Design review of the part built by this model. Coordinates are the model's own, in mm. A direction names the side the tool comes from. Coordinates: 2 decimals unless noted, no trailing zeros. Write each loop counter-clockwise with the first axis right and the second up, starting at its lowest first coordinate (ties: lowest second). Pieces come first, ordered by that corner, then holes.
```python
from build123d import *

# Parameters (mm, degrees)
SKETCH1_W                       = 40.894
SKETCH1_H                       = 25.4
REVOLVE1_ANGLE                  = 180
BOSS_EXTRUDE1_REACH             = 27.4
SKETCH3_W                       = 25.654
SKETCH3_H                       = 4.572
BOSS_EXTRUDE1_DIRECTION_2_REACH = 27.4
SKETCH4_W                       = 25.654
SKETCH4_H                       = 24.524924672
CUT_EXTRUDE1_DEPTH              = 4.572
SKETCH5_W                       = 3.81
SKETCH5_H                       = 2.032
BOSS_EXTRUDE2_DEPTH             = 25.654


with BuildPart() as part:
    # Sketch1 → Revolve1 (revolve)
    with BuildSketch(Plane(origin=(0, 0, 0), x_dir=(1, 0, 0), z_dir=(0, 1, 0))):
        with Locations((20.447, -12.7)):
            Rectangle(SKETCH1_W, SKETCH1_H)
    revolve(axis=Axis((0, 0, 0), (1, 0, 0)), revolution_arc=REVOLVE1_ANGLE)

    # Sketch2 → Cut-Revolve1 (revolve, cut)
    with BuildSketch(Plane(origin=(0, 0, 0), x_dir=(1, 0, 0), z_dir=(0, 1, 0))):
        Polygon((0, 0), (41.402, 0), (41.402, -20.701), (40.132, -20.701), (1.27, -20.701), (0, -20.701), align=None)
    revolve(axis=Axis((0, 0, 0), (1, 0, 0)), mode=Mode.SUBTRACT)

    # Sketch3 → Boss-Extrude1 (add, up to next)
    with BuildSketch(Plane.XY, mode=Mode.PRIVATE) as boss_extrude1_sk1:
        with Locations((20.447, -13.97)):
            Rectangle(SKETCH3_W, SKETCH3_H)
    boss_extrude1_tool1 = extrude(boss_extrude1_sk1.sketch, amount=BOSS_EXTRUDE1_REACH, mode=Mode.PRIVATE) - part.part
    add(boss_extrude1_tool1.solids().sort_by_distance((20.447, -13.97, 0))[0])

    # Sketch3 → Boss-Extrude1 direction 2 (add, up to next)
    with BuildSketch(Plane.XY, mode=Mode.PRIVATE) as boss_extrude1_direction_2_sk1:
        with Locations((20.447, -13.97)):
            Rectangle(SKETCH3_W, SKETCH3_H)
    boss_extrude1_direction_2_tool1 = extrude(boss_extrude1_direction_2_sk1.sketch, amount=-BOSS_EXTRUDE1_DIRECTION_2_REACH, mode=Mode.PRIVATE) - part.part
    add(boss_extrude1_direction_2_tool1.solids().sort_by_distance((20.447, -13.97, 0))[0])

    # Sketch4 → Cut-Extrude1 (cut)
    with BuildSketch(Plane(origin=(0, -11.684, 0), x_dir=(1, 0, 0), z_dir=(0, 1, 0))):
        with Locations((20.447, 0)):
            Rectangle(SKETCH4_W, SKETCH4_H)
    extrude(amount=-CUT_EXTRUDE1_DEPTH, mode=Mode.SUBTRACT)

    # Sketch5 → Boss-Extrude2 (add)
    with BuildSketch(Plane.ZY.offset(-7.62)):
        with Locations((-10.357462336, -13.97)):
            Rectangle(SKETCH5_W, SKETCH5_H)
        with Locations((10.357462336, -13.97)):
            Rectangle(SKETCH5_W, SKETCH5_H)
    extrude(amount=-BOSS_EXTRUDE2_DEPTH)


solid = part.part
```
(1) Wall thickness on line 1 (Z direction, x = 19, y = -6.75); line 2 (Y direction, x = 18, z = -11); line 3 (Z direction, x = 3, y = -8.75): over which ranges is each line inside the solid? List them lowest first.
(2) Consider section B-B (y = -10). Give the boundary of the cut face in (x, z), plus the area to 3 significant figures.
(3) Consider section C-C (z = -16). Give the boundary of the cut face in (x, y).
(4) Consider section A-A (x = 32). Give the boundary of the cut face in (y, z).
(5) For faces 1 (the flat face through (33.274, -13, 13)), 2 (the flat face through (20, -14, -8.452)), 3 (the flat face through (7.62, -13, -13)), list the 3-axis set-ups (+Z, -Z, +X, -X, +Y, -Y) from which the entire face can be reached by the end or side of a thin tool; tool diameter is ignored.
(6) Consider section D-D (z = 0). Give the boundary of the cut face in (x, y).
(7) Mouldability with a two-part tool opening along Y and no side actions: class faces 4 (the flat face through (20, -11.684, 15)), 5 (the flat face through (20, -14, 8.452)), 6 (the flat face through (20, -16, 12.262)) as +Y half, -Y half, draft (parallel to the pull), parting line (faces both ways), or undercut.
(8) Insertion check: pin 1 Ø1 at (x, y) = (14, -12.5) entering from -Z; pin 2 Ø1.4 at (x, z) = (25, -16) entering from +Y; pin 3 Ø1.1 at (x, z) = (21.5, 10.5) entering from -Y; pin 4 Ø3.5 at (y, z) = (-13, 15) entering from -X. Each pin has a flat end and moves straight along its axis. Give the tip position at first contact, or say it passes through.
Results:
1. line 1: z = -24.49 to -19.57, 19.57 to 24.49
1. line 2: y = -22.89 to -17.54, -14.99 to -12.95
1. line 3: z = -23.85 to -18.76, 18.76 to 23.85
2. outline: (0, -23.35) - (40.89, -23.35) - (40.89, -18.13) - (0, -18.13) - close; (0, 18.13) - (40.89, 18.13) - (40.89, 23.35) - (0, 23.35) - close
2. area: 427 mm2
3. outline: (0, -19.73) - (40.89, -19.73) - (40.89, -13.14) - (33.27, -13.14) - (33.27, -11.68) - (7.62, -11.68) - (7.62, -13.14) - (0, -13.14) - close
4. outline: (-16.26, -12.82) arc R20.7 cw to (-16.26, 12.82) - (-16.26, 12.26) - (-14.99, 12.26) - (-14.99, 8.45) - (-12.95, 8.45) - (-12.95, 12.26) - (-11.68, 12.26) - (-11.68, 17.09) arc R20.7 cw to (0, 20.7) - (0, 25.4) arc R25.4 ccw to (0, -25.4) - (0, -20.7) arc R20.7 cw to (-11.68, -17.09) - (-11.68, -12.26) - (-12.95, -12.26) - (-12.95, -8.45) - (-14.99, -8.45) - (-14.99, -12.26) - (-16.26, -12.26) - close
5. face 1: +X, +Y
5. face 2: +X, -X, +Y
5. face 3: -X, +Y
6. outline: (0, -25.4) - (40.89, -25.4) - (40.89, -20.7) - (0, -20.7) - close
7. face 4: +Y half
7. face 5: draft
7. face 6: undercut
8. pin 1: stops at z = -22.39
8. pin 2: stops at y = -11.68
8. pin 3: stops at y = -23.37
8. pin 4: stops at x = 0
